Read the model definition and answer for the solid it produces. Units are mm, in the model's axes. Face numbers are marked on the shaded views. A direction names the side the tool comes from. Give positions to 0.01 mm unless a question says otherwise; leave off trailing zeros. Order: outer loops, then holes, each group sorted by start corner. A loop starts at its lowest first (then second) coordinate and runs counter-clockwise, first axis right, second up. Notation, with made-up numbers: (-20, 32) - (18, 32) arc R10 cw to (18, 48) - close; hole circle Ø6 at (63, -12). An arc over 180 degrees is marked (long way). Return JSON: item names as keys, results as strings.
```python
from build123d import *

# Parameters (mm, degrees)
BOSS_EXTRUDE1_DEPTH = 70
SHELL1_T            = -3
SKETCH5_W           = 100
SKETCH5_H           = 80
CUT_EXTRUDE2_DEPTH  = 30
FILLET1_R           = 10
FILLET2_R           = 3


with BuildPart() as part:
    # Sketch3 → Boss-Extrude1 (new body)
    with BuildSketch(Plane(origin=(0, 0, 0), x_dir=(1, 0, 0), z_dir=(0, 1, 0))):
        Polygon((0, 330.560430114), (-233.741521725, 233.741521725), (-330.560430114, 0), (-233.741521725, -233.741521725), (0, -330.560430114), (233.741521725, -233.741521725), (330.560430114, 0), (233.741521725, 233.741521725), align=None)
    extrude(amount=BOSS_EXTRUDE1_DEPTH)

    # Shell1
    shell1_openings = [part.faces().sort_by_distance(p)[0] for p in [
        (0, 0, 0),
    ]]
    offset(amount=SHELL1_T, openings=shell1_openings, kind=Kind.INTERSECTION)

    # Sketch5 → Cut-Extrude2 (cut)
    with BuildSketch(Plane(origin=(331, 0, 0), x_dir=(0, 0, -1), z_dir=(1, 0, 0))):
        with Locations((0, 40)):
            Rectangle(SKETCH5_W, SKETCH5_H)
    extrude(amount=-CUT_EXTRUDE2_DEPTH, mode=Mode.SUBTRACT)

    # Fillet1
    fillet1_edges = [part.edges().sort_by_distance(p)[0] for p in [
        (271.79563686, 70, 141.870760863),
        (116.870760863, 70, 282.15097592),
        (-116.870760863, 70, 282.15097592),
        (-282.15097592, 70, 116.870760863),
        (-282.15097592, 70, -116.870760863),
        (-116.870760863, 70, -282.15097592),
        (116.870760863, 70, -282.15097592),
        (271.79563686, 70, -141.870760863),
    ]]
    fillet(fillet1_edges, radius=FILLET1_R)

    # Fillet2
    fillet2_edges = [part.edges().sort_by_distance(p)[0] for p in [
        (115.722710566, 67, 279.379337322),
        (269.023998263, 67, 140.722710566),
        (115.722710566, 67, -279.379337322),
        (-115.722710566, 67, -279.379337322),
        (-279.379337322, 67, -115.722710566),
        (-279.379337322, 67, 115.722710566),
        (-115.722710566, 67, 279.379337322),
        (269.023998263, 67, -140.722710566),
    ]]
    fillet(fillet2_edges, radius=FILLET2_R)


solid = part.part
```
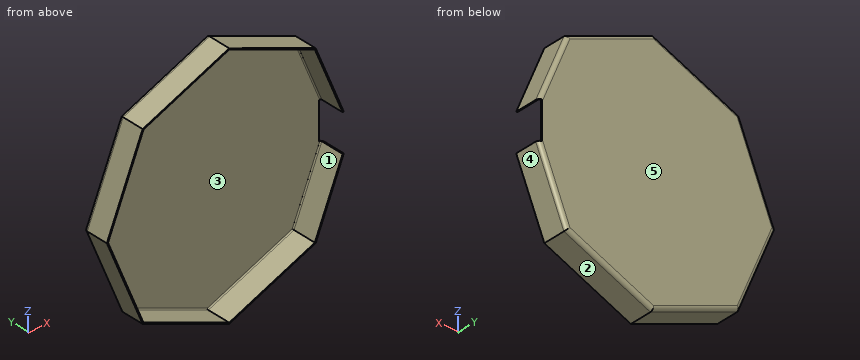
Q1. Determine the mould class of the marked faces 3, 4 and 5 for opening direction Z: released by +Z, released by -Z, zero draft, split by the parting line, or undercut.
Values:
{"face 3": "undercut", "face 4": "released by -Z", "face 5": "zero draft"}
Q2. Given pin 1 (3 mm diameter, centred on x = 29, z = 154.5, fed in from -Y); pin 2 (5 mm diameter, centred on y = 62.5, z = -218, fed in from +X); pin 3 (6 mm diameter, centred on x = -157, y = 12.5, fed in from +Z), each flat-ended and moving along its own axis, determine where each tip first touches the part or whether it passes through.
Values:
{"pin 1": "stops at y = 67", "pin 2": "stops at x = 241.09", "pin 3": "stops at z = 266.77"}
Q3. For the marked faces 1 and 2, determine the directions among +Z, -Z, +X, -X, +Y, -Y from which every point of the face is accessible in a straight line to the end or side of a thin tool.
Values:
{"face 1": "-Y", "face 2": "-Z, +X, +Y, -Y"}
Q4. Consider L1, parallel to Z at x = -7.5, y = 19; L2, parallel to X at y = 49, z = 264; L3, parallel to X at y = 11, z = 204. Determine where each line is inside the solid, lowest interval first.
Values:
{"L1": "z = -327.45 to -324.21, 324.21 to 327.45", "L2": "x = -160.69 to -152.85, 152.85 to 160.69", "L3": "x = -246.06 to -242.81, 242.81 to 246.06"}
Q5. A cutting plane is placed at A-A (y = 47). Write down the section's boundary in (x, z).
Values:
{"outline": "(-330.56, 0) - (-233.74, -233.74) - (0, -330.56) - (233.74, -233.74) - (309.85, -50) - (306.6, -50) - (231.45, -231.45) - (0, -327.31) - (-231.45, -231.45) - (-327.31, 0) - (-231.45, 231.45) - (0, 327.31) - (231.45, 231.45) - (306.6, 50) - (309.85, 50) - (233.74, 233.74) - (0, 330.56) - (-233.74, 233.74) - close"}
